Model file for the job. Use its own axes, mm. A direction names the side the tool comes from. Coordinates: 2 decimals unless noted, no trailing zeros. Loops run counter-clockwise (first coordinate to the right, second up) from the corner with the lowest first, then second, coordinate; pieces in that order, holes last. Notation, with made-up numbers: M 60,63.5 L 78,63.5 A21 cw 78,85.5 Z; hole C 17,17 d3. An arc over 180 degrees is marked long. Write item = value, one per line. Start each with the question number.
from build123d import *

# Parameters (mm, degrees)
FRONT_START        = 0.495634701
FRONT_PLATE_DEPTH  = 2.95
SKETCH1_W          = 5
SKETCH1_H          = 5.3
CUT_EXTRUDE2_DEPTH = 98.689964927
CUT_EXTRUDE3_START = 2.95
SKETCH3_W          = 3.2
SKETCH3_H          = 3.2
CUT_EXTRUDE3_DEPTH = 12
SKETCH4_W          = 2.3
SKETCH4_H          = 5.3
CUT_EXTRUDE4_DEPTH = 98.689964927


# Read off the part's stored shape, not the designer's step: Front Plate
with BuildPart() as part:
    # Front Plate outline → Front Plate (new body)
    with BuildSketch(Plane.YZ.offset(FRONT_START)):
        Polygon((-18.627257495, 18.295409887), (-7.556257495, 18.295409887), (-7.556257495, 30.360409887), (-4.606257495, 30.360409887), (-4.606257495, 18.295409887), (-6.352257495, 18.295409887), (-6.352257495, 15.345409887), (3.647742505, 15.345409887), (3.647742505, 18.295409887), (13.647742505, 18.295409887), (13.647742505, 15.345409887), (23.647742505, 15.345409887), (23.647742505, 18.295409887), (33.647742505, 18.295409887), (33.647742505, 15.345409887), (43.647742505, 15.345409887), (43.647742505, 18.295409887), (53.647742505, 18.295409887), (53.647742505, 15.345409887), (63.647742505, 15.345409887), (63.647742505, 18.295409887), (61.901742505, 18.295409887), (61.901742505, 30.360409887), (64.851742505, 30.360409887), (64.851742505, 18.295409887), (75.922742505, 18.295409887), (75.922742505, 23.045409887), (74.872742505, 23.045409887), (74.872742505, 25.345409887), (75.922742505, 25.345409887), (75.922742505, 27.345409887), (79.122742505, 27.345409887), (79.122742505, 25.345409887), (80.172742505, 25.345409887), (80.172742505, 23.045409887), (79.122742505, 23.045409887), (79.122742505, 18.295409887), (83.647742505, 18.295409887), (83.647742505, 47.425409887), (63.647742505, 47.425409887), (63.647742505, 50.375409887), (53.647742505, 50.375409887), (53.647742505, 47.425409887), (43.647742505, 47.425409887), (43.647742505, 50.375409887), (33.647742505, 50.375409887), (33.647742505, 47.425409887), (23.647742505, 47.425409887), (23.647742505, 50.375409887), (13.647742505, 50.375409887), (13.647742505, 47.425409887), (3.647742505, 47.425409887), (3.647742505, 50.375409887), (-6.352257495, 50.375409887), (-6.352257495, 47.425409887), (-26.352257495, 47.425409887), (-26.352257495, 18.295409887), (-21.827257495, 18.295409887), (-21.827257495, 23.045409887), (-22.877257495, 23.045409887), (-22.877257495, 25.345409887), (-21.827257495, 25.345409887), (-21.827257495, 27.345409887), (-18.627257495, 27.345409887), (-18.627257495, 25.345409887), (-17.577257495, 25.345409887), (-17.577257495, 23.045409887), (-18.627257495, 23.045409887), align=None)
    extrude(amount=FRONT_PLATE_DEPTH)

    # Sketch1 → Cut-Extrude2 (cut, through all)
    with BuildSketch(Plane(origin=(3.445634701, 0, 0), x_dir=(0, 0, -1), z_dir=(1, 0, 0))):
        with Locations((-44.925409887, -20.227257495)):
            Rectangle(SKETCH1_W, SKETCH1_H)
    cut_extrude2 = extrude(amount=-CUT_EXTRUDE2_DEPTH, mode=Mode.SUBTRACT)

    # Sketch3 → Cut-Extrude3 (cut)
    with BuildSketch(Plane.XY.offset(47.425409887).offset(CUT_EXTRUDE3_START)):
        with Locations((1.970634701, 8.647742505)):
            Rectangle(SKETCH3_W, SKETCH3_H)
    cut_extrude3 = extrude(amount=-CUT_EXTRUDE3_DEPTH, mode=Mode.SUBTRACT)

    # Sketch4 → Cut-Extrude4 (cut, through all)
    with BuildSketch(Plane(origin=(3.445634701, 0, 0), x_dir=(0, 0, -1), z_dir=(1, 0, 0))):
        with Locations((-41.525409887, 8.647742505)):
            Rectangle(SKETCH4_W, SKETCH4_H)
    cut_extrude4 = extrude(amount=-CUT_EXTRUDE4_DEPTH, mode=Mode.SUBTRACT)

    # Mirror1: Cut-Extrude2, Cut-Extrude3, Cut-Extrude4 across plane
    add(cut_extrude2.mirror(Plane.ZX.offset(28.647742505)), mode=Mode.SUBTRACT)
    add(cut_extrude3.mirror(Plane.ZX.offset(28.647742505)), mode=Mode.SUBTRACT)
    add(cut_extrude4.mirror(Plane.ZX.offset(28.647742505)), mode=Mode.SUBTRACT)


solid = part.part
Item 1: Cut at B-B (y = -14.5). Give the cut face in (x, z).
Item 2: Pull direction Z, two halves, no side cores. Call faces 1 (the flat face through (2, 74.873, 45)), 2 (the flat face through (2, 45, 47.425)), 3 (the flat face through (2, 45.998, 42)): +Z half, -Z half, draft (parallel to the pull), parting line (faces both ways), or undercut.
Item 3: Probe L1, parallel to Y at x = 0.9, z = 40.5; L2, parallel to Y at x = 1.35, z = 24; L3, parallel to Y at x = 3.05, z = 17. List the from-to ranges inside material, lowest first.
Item 4: Cut at C-C (y = 8). Give the cut face in (x, z), plus the area to 3 significant figures.
Item 5: 3-axis set-ups, long thin cutter, end or side, ignore diameter. For faces 4 (the flat face through (2, 61.902, 24)), 5 (the flat face through (2, 81, 18.295)), 6 (the flat face through (2, 33.648, 17)): which of +Z, -Z, +X, -X, +Y, -Y reach the whole face in a straight line?
Item 6: Cut at A-A (z = 24). Give the cut face in (x, y).
Item 7: Pin check, flat tips, straight feed: pin 1 Ø1.5 at (x, y) = (2.5, 5) entering from +Z; pin 2 Ø0.9 at (x, y) = (2.5, 78) entering from -Z; pin 3 Ø0.8 at (x, y) = (2.5, 75.5) entering from +Z. Stop position of each tip, or through.
Reported:
q1.outline = M 0.5,18.3 L 3.45,18.3 L 3.45,47.43 L 0.5,47.43 Z
q2.face_1 = draft
q2.face_2 = +Z half
q2.face_3 = undercut
q3.L1 = -26.35 to 6, 11.3 to 46, 51.3 to 83.65
q3.L2 = -26.35 to -22.88, -17.58 to -7.56, -4.61 to 61.9, 64.85 to 74.87, 80.17 to 83.65
q3.L3 = -6.35 to 3.65, 13.65 to 23.65, 33.65 to 43.65, 53.65 to 63.65
q4.outline = M 0.5,18.3 L 3.45,18.3 L 3.45,38.38 L 0.5,38.38 Z
q4.area = 59.2 mm^2
q5.face_4 = +X, -X
q5.face_5 = -Z, +X, -X, +Y
q5.face_6 = -Z, +X, -X
q6.outline = M 0.5,-26.35 L 3.45,-26.35 L 3.45,-22.88 L 0.5,-22.88 Z; M 0.5,-17.58 L 3.45,-17.58 L 3.45,-7.56 L 0.5,-7.56 Z; M 0.5,-4.61 L 3.45,-4.61 L 3.45,61.9 L 0.5,61.9 Z; M 0.5,64.85 L 3.45,64.85 L 3.45,74.87 L 0.5,74.87 Z; M 0.5,80.17 L 3.45,80.17 L 3.45,83.65 L 0.5,83.65 Z
q7.pin_1 = 47.43
q7.pin_2 = 27.35
q7.pin_3 = 42.43
